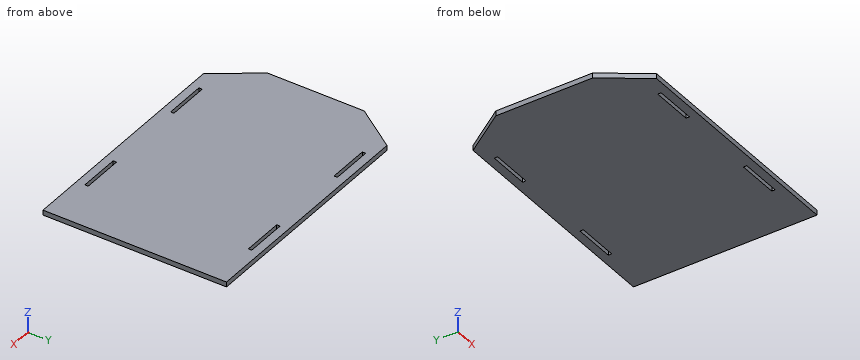
from build123d import *

# Parameters (mm, degrees)
SKIZZE1_W                       = 320
SKIZZE1_H                       = 220
AUFSATZ_LINEAR_AUSTRAGEN1_DEPTH = 6
SKIZZE2_W                       = 50
SKIZZE2_H                       = 4
SCHNITT_LINEAR_AUSTRAGEN1_DEPTH = 6
SPIEGELN2_COPY_1_SKETCH_W       = 50
SPIEGELN2_COPY_1_SKETCH_H       = 4
SPIEGELN2_COPY_1_DEPTH          = 6
SCHNITT_LINEAR_AUSTRAGEN2_DEPTH = 6


with BuildPart() as part:
    # Skizze1 → Aufsatz-Linear austragen1 (new body)
    with BuildSketch(Plane.XY):
        with Locations((160, 110)):
            Rectangle(SKIZZE1_W, SKIZZE1_H)
    extrude(amount=AUFSATZ_LINEAR_AUSTRAGEN1_DEPTH)

    # Skizze2 → Schnitt-Linear austragen1 (cut)
    with BuildSketch(Plane.XY.offset(6)):
        with Locations((84.3, 208)):
            Rectangle(SKIZZE2_W, SKIZZE2_H)
    schnitt_linear_austragen1 = extrude(amount=-SCHNITT_LINEAR_AUSTRAGEN1_DEPTH, mode=Mode.SUBTRACT)

    # Spiegeln1: Schnitt-Linear austragen1 across plane
    add(schnitt_linear_austragen1.mirror(Plane(origin=(160, 0, 0), x_dir=(0, 0, 1), z_dir=(1, 0, 0))), mode=Mode.SUBTRACT)

    # Spiegeln2: Schnitt-Linear austragen1 across plane
    add(schnitt_linear_austragen1.mirror(Plane.ZX.offset(110)), mode=Mode.SUBTRACT)

    # Spiegeln2 copy 1 sketch → Spiegeln2 copy 1 (cut)
    with BuildSketch(Plane(origin=(320, 220, 6), x_dir=(-1, 0, 0), z_dir=(0, 0, 1))):
        with Locations((84.3, 208)):
            Rectangle(SPIEGELN2_COPY_1_SKETCH_W, SPIEGELN2_COPY_1_SKETCH_H)
    extrude(amount=-SPIEGELN2_COPY_1_DEPTH, mode=Mode.SUBTRACT)

    # Skizze3 → Schnitt-Linear austragen2 (cut)
    with BuildSketch(Plane.XY.offset(6)):
        Polygon((0, 52), (36.410791987, 0), (0, 0), align=None)
    schnitt_linear_austragen2 = extrude(amount=-SCHNITT_LINEAR_AUSTRAGEN2_DEPTH, mode=Mode.SUBTRACT)

    # Spiegeln3: Schnitt-Linear austragen2 across plane
    add(schnitt_linear_austragen2.mirror(Plane.ZX.offset(110)), mode=Mode.SUBTRACT)


solid = part.part
Read the model definition and answer for the solid it produces. Units are mm, in the model's axes. Round coordinates to 2 decimals unless told otherwise and drop trailing zeros. Loops run counter-clockwise (first coordinate to the right, second up) from the corner with the lowest first, then second, coordinate; pieces in that order, holes last.
Q1. Section D-D on y = 175 is taken. Write down the section's boundary in (x, z).
Q2. Consider probe 1 along Y at (x, z) = (260.5, 2.85); probe 2 along X at (y, z) = (176.5, 0.5); probe 3 along Y at (x, z) = (27, 0.55). Determine where each line is inside the solid, lowest interval first.
Q3. Section C-C on y = 27 is taken. Write down the section's boundary in (x, z).
Q4. Section B-B on x = 67 is taken. Write down the section's boundary in (y, z), and give its area (3 significant figures).
Q5. Each of these flat-tipped pins is pushed along its axis until it touches: pin 1 (10 mm diameter, centred on x = 266, y = 126.5, fed in from -Z); pin 2 (2 mm diameter, centred on y = 207.5, z = 2.5, fed in from -X); pin 3 (2 mm diameter, centred on y = 207, z = 3.5, fed in from -X); pin 4 (2 mm diameter, centred on y = 11, z = 3.5, fed in from -X). Where does it stop, or does it pass through?
Q6. Section A-A on z = 1.15 is taken. Write down the section's boundary in (x, y), and give its area (3 significant figures).
Output:
1. outline: (4.9, 0) - (320, 0) - (320, 6) - (4.9, 6) - close
2. probe 1: y = 0 to 10, 14 to 206, 210 to 220
2. probe 2: x = 5.95 to 320
2. probe 3: y = 13.44 to 206.56
3. outline: (17.51, 0) - (320, 0) - (320, 6) - (17.51, 6) - close
4. outline: (0, 0) - (10, 0) - (10, 6) - (0, 6) - close; (14, 0) - (206, 0) - (206, 6) - (14, 6) - close; (210, 0) - (220, 0) - (220, 6) - (210, 6) - close
4. area: 1,270 mm2
5. pin 1: stops at z = 0
5. pin 2: stops at x = 26.96
5. pin 3: stops at x = 26.61
5. pin 4: stops at x = 28.01
6. outline: (0, 52) - (36.41, 0) - (320, 0) - (320, 220) - (36.41, 220) - (0, 168) - close; hole (59.3, 10) - (109.3, 10) - (109.3, 14) - (59.3, 14) - close; hole (59.3, 206) - (109.3, 206) - (109.3, 210) - (59.3, 210) - close; hole (210.7, 10) - (260.7, 10) - (260.7, 14) - (210.7, 14) - close; hole (210.7, 206) - (260.7, 206) - (260.7, 210) - (210.7, 210) - close
6. area: 67,700 mm2
